Read the model definition and answer for the solid it produces. Units are mm, in the model's axes. A direction names the side the tool comes from. Round coordinates to 2 decimals unless told otherwise and drop trailing zeros. Write each loop counter-clockwise with the first axis right and the second up, starting at its lowest first coordinate (ties: lowest second). Pieces come first, ordered by that corner, then holes. Notation, with made-up numbers: (31, -33) - (54, -33) arc R25 ccw to (54, -7) - close; hole circle Ø1 at (-36.75, -4.5). An arc over 180 degrees is marked (long way). Answer as CSV lines item,"result". Start each with the question number.
1) Find section C-C on y = -20. Determine the outline of the cut face in (x, z).
2) Which of the six approach directions +Z, -Z, +X, -X, +Y, -Y give full straight-line access (tool end or side, diameter ignored) to faces 4 (the flat face through (81, -15, 2)), 5 (the flat face through (0, -25, 66))?
3) This flat-tipped pin is pushed along its axis until it touches: pin 1 (1.6 mm diameter, centred on x = 89.5, z = 0.5, fed in from +Y). Where does it stop, or does it pass through?
4) For a pull along X with two mould halves and no side action, classify faces 1 (the flat face through (81, -15, 0)), 2 (the flat face through (162, -25, 66)), 3 (the flat face through (164, -25, 66)) as +X half, -X half, draft (parallel to the pull), parting line (faces both ways), or undercut.
5) Consider line 1 along X through (y, z) = (-35.5, 19.5); line 2 along Z through (x, y) = (96, -10). Determine where each line is inside the solid, lowest interval first.
6) Find section D-D on z = 119.5. Determine the outline of the cut face in (x, y), then the cut area to 3 significant figures.
7) Find section A-A on x = 63.5. Determine the outline of the cut face in (y, z).
8) Find section B-B on z = 96. Determine the outline of the cut face in (x, y), then the cut area to 3 significant figures.
from build123d import *

# Parameters (mm, degrees)
ESQUISSE1_W             = 164
ESQUISSE1_H             = 40
BOSS_EXTRU_1_DEPTH      = 2
ESQUISSE2_W             = 2
ESQUISSE2_H             = 40
BOSS_EXTRU_2_DEPTH      = 130
ESQUISSE3_W             = 2
ESQUISSE3_H             = 40
BOSS_EXTRU_3_DEPTH      = 130
ESQUISSE4_R             = 2
ENL_V_MAT_EXTRU_1_DEPTH = 165
CONG_1_R                = 1
CONG_2_R                = 1
ESQUISSE5_W             = 75
ESQUISSE5_H             = 6
ENL_V_MAT_EXTRU_2_DEPTH = 130
ENL_V_MAT_EXTRU_3_DEPTH = 165


with BuildPart() as part:
    # Esquisse1 → Boss.-Extru.1 (new body)
    with BuildSketch(Plane.XY):
        with Locations((82, -20)):
            Rectangle(ESQUISSE1_W, ESQUISSE1_H)
    extrude(amount=BOSS_EXTRU_1_DEPTH)

    # Esquisse2 → Boss.-Extru.2 (add)
    with BuildSketch(Plane.XY.offset(2)):
        with Locations((1, -20)):
            Rectangle(ESQUISSE2_W, ESQUISSE2_H)
    extrude(amount=BOSS_EXTRU_2_DEPTH)

    # Esquisse3 → Boss.-Extru.3 (add)
    with BuildSketch(Plane.XY.offset(2)):
        with Locations((163, -20)):
            Rectangle(ESQUISSE3_W, ESQUISSE3_H)
    extrude(amount=BOSS_EXTRU_3_DEPTH)

    # Esquisse4 → Enlèv. mat.-Extru.1 (cut, through all)
    with BuildSketch(Plane.ZY):
        with Locations((112, -20)):
            Circle(ESQUISSE4_R)
    extrude(amount=-ENL_V_MAT_EXTRU_1_DEPTH, mode=Mode.SUBTRACT)

    # Congé1
    cong_1_edges = [part.edges().sort_by_distance(p)[0] for p in [
        (0, -20, 0),
    ]]
    fillet(cong_1_edges, radius=CONG_1_R)

    # Congé2
    cong_2_edges = [part.edges().sort_by_distance(p)[0] for p in [
        (164, -20, 0),
    ]]
    fillet(cong_2_edges, radius=CONG_2_R)

    # Esquisse5 → Enlèv. mat.-Extru.2 (cut)
    with BuildSketch(Plane.XY.offset(2)):
        with Locations((82, -20)):
            Rectangle(ESQUISSE5_W, ESQUISSE5_H)
    extrude(amount=-ENL_V_MAT_EXTRU_2_DEPTH, mode=Mode.SUBTRACT)

    # Esquisse6 → Enlèv. mat.-Extru.3 (cut, through all)
    with BuildSketch(Plane.ZY):
        with BuildLine():
            Line((62, -18), (112, -18))
            ThreePointArc((112, -18), (114, -20), (112, -22))
            Line((112, -22), (62, -22))
            ThreePointArc((62, -22), (60, -20), (62, -18))
        make_face()
    extrude(amount=-ENL_V_MAT_EXTRU_3_DEPTH, mode=Mode.SUBTRACT)


solid = part.part
Check values:
1,outline,"(0, 1) arc R1 ccw to (1, 0) - (44.5, 0) - (44.5, 2) - (2, 2) - (2, 60) - (0, 60) - close; (0, 114) - (2, 114) - (2, 132) - (0, 132) - close; (119.5, 0) - (163, 0) arc R1 ccw to (164, 1) - (164, 60) - (162, 60) - (162, 2) - (119.5, 2) - close; (162, 114) - (164, 114) - (164, 132) - (162, 132) - close"
2,face 4,"+Z, +Y, -Y"
2,face 5,"+Z, -Z, -X, +Y, -Y"
3,pin 1,"stops at y = 0"
4,face 1,"draft"
4,face 2,"undercut"
4,face 3,"+X half"
5,line 1,"x = 0 to 2, 162 to 164"
5,line 2,"z = 0 to 2"
6,outline,"(0, -40) - (2, -40) - (2, 0) - (0, 0) - close; (162, -40) - (164, -40) - (164, 0) - (162, 0) - close"
6,area,"160 mm^2"
7,outline,"(-40, 0) - (-23, 0) - (-23, 2) - (-40, 2) - close; (-17, 0) - (0, 0) - (0, 2) - (-17, 2) - close"
8,outline,"(0, -40) - (2, -40) - (2, -22) - (0, -22) - close; (0, -18) - (2, -18) - (2, 0) - (0, 0) - close; (162, -40) - (164, -40) - (164, -22) - (162, -22) - close; (162, -18) - (164, -18) - (164, 0) - (162, 0) - close"
8,area,"144 mm^2"
